from build123d import *

# Parameters (mm, degrees)
SKETCH1_R           = 5
BOSS_EXTRUDE1_DEPTH = 8
SKETCH2_R           = 5
BOSS_EXTRUDE2_DEPTH = 2
BOSS_EXTRUDE3_DEPTH = 10


with BuildPart() as part:
    # Sketch1 → Boss-Extrude1 (new body)
    with BuildSketch(Plane(origin=(0, 0, 0), x_dir=(1, 0, 0), z_dir=(0, 1, 0))):
        Circle(SKETCH1_R)
        with BuildLine():
            Line((-2, 1.5), (2, 1.5))
            ThreePointArc((2, 1.5), (0, -2.5), (-2, 1.5))
        make_face(mode=Mode.SUBTRACT)
    extrude(amount=BOSS_EXTRUDE1_DEPTH)

    # Sketch2 → Boss-Extrude2 (add)
    with BuildSketch(Plane(origin=(0, 8, 0), x_dir=(1, 0, 0), z_dir=(0, 1, 0))):
        Circle(SKETCH2_R)
    extrude(amount=BOSS_EXTRUDE2_DEPTH)

    # Sketch3 → Boss-Extrude3 (add)
    with BuildSketch(Plane(origin=(0, 10, 0), x_dir=(1, 0, 0), z_dir=(0, 1, 0))):
        with BuildLine():
            Line((-1.609347694, 1.5), (1.609347694, 1.5))
            ThreePointArc((1.609347694, 1.5), (2.2, 0), (1.609347694, -1.5))
            Line((1.609347694, -1.5), (-1.609347694, -1.5))
            ThreePointArc((-1.609347694, -1.5), (-2.2, 0), (-1.609347694, 1.5))
        make_face()
    extrude(amount=BOSS_EXTRUDE3_DEPTH)


solid = part.part
CAD build for the part. Positions are in the model's coordinates, mm. A direction names the side the tool comes from. Give positions to 0.01 mm unless a question says otherwise; leave off trailing zeros. Order: outer loops, then holes, each group sorted by start corner. A loop starts at its lowest first (then second) coordinate and runs counter-clockwise, first axis right, second up. Notation, with made-up numbers: (-26.75, 29.5) -> (-10.75, 29.5) arc R16 ccw to (-10.75, 45.5) -> close; hole circle Ø8 at (7.25, 24). An arc over 180 degrees is marked (long way). Return JSON: item names as keys, results as strings.
Q1. Which spindle directions (+Z, -Z, +X, -X, +Y, -Y) get a long thin tool onto all of the face, cutting with end or side? Do faces 1 (the face through (-2.2, 14.9, 0)), 2 (the face through (2.2, 14.9, 0)), 3 (the face through (0, 4, -1.5)), 4 (the face through (0, 10, 2)). Say none if no direction does.
Working result:
{"face 1": "-X, +Y", "face 2": "+X, +Y", "face 3": "-Y", "face 4": "+Y"}
Q2. Flat gauge pins, fed straight in: pin 1 (1 mm diameter, centred on x = 2.5, y = 10, fed in from -Z); pin 2 (1.5 mm diameter, centred on y = 11, z = 2, fed in from -X); pin 3 (5 mm diameter, centred on y = 6.5, z = -3.5, fed in from -X). Where does each tip first touch, or does it go through?
Working result:
{"pin 1": "z = -4.58", "pin 2": "x = -1.81", "pin 3": "x = -4.9"}
Q3. Saw through at A-A (z = 0). Write the cut outline in (x, y), then the cut area to 3 significant figures.
Working result:
{"outline": "(-5, 0) -> (-2.5, 0) -> (-2.5, 8) -> (2.5, 8) -> (2.5, 0) -> (5, 0) -> (5, 10) -> (2.2, 10) -> (2.2, 20) -> (-2.2, 20) -> (-2.2, 10) -> (-5, 10) -> close", "area": "104 mm²"}
Q4. Saw through at B-B (x = 0). Write the cut outline in (y, z).
Working result:
{"outline": "(0, -5) -> (10, -5) -> (10, -1.5) -> (20, -1.5) -> (20, 1.5) -> (10, 1.5) -> (10, 5) -> (0, 5) -> (0, 2.5) -> (8, 2.5) -> (8, -1.5) -> (0, -1.5) -> close"}
Q5. Saw through at C-C (y = 13.75). Write the cut outline in (x, z).
Working result:
{"outline": "(-1.61, -1.5) -> (1.61, -1.5) arc R2.2 ccw to (1.61, 1.5) -> (-1.61, 1.5) arc R2.2 ccw to start"}
Q6. Mould opens along Z. For faces 5 (the face through (0, 15, -1.5)), 6 (the face through (0, 0, -2)), 7 (the face through (0, 15, 1.5)), 8 (the face through (0, 8, 0)) say: pulls with the +Z half, pulls with the -Z half, needs draft (parallel to the pull), parting line crosses it, or undercut.
Working result:
{"face 5": "pulls with the -Z half", "face 6": "needs draft", "face 7": "pulls with the +Z half", "face 8": "undercut"}
Q7. Saw through at D-D (y = 3.25). Write the cut outline in (x, z).
Working result:
{"outline": "circle Ø10 at (0, 0); hole (-2, -1.5) -> (2, -1.5) arc R2.5 ccw (long way) to start"}
Q8. Drill centre lines: line 1 (X direction, y = 4.25, z = 0); line 2 (Z direction, x = 0.75, y = 11.5); line 3 (Y direction, x = -2, z = 3.5). Where is each one in solid material? Low to high.
Working result:
{"line 1": "-5 to -2.5, 2.5 to 5", "line 2": "-1.5 to 1.5", "line 3": "0 to 10"}
